Source: CAD feature listing. Evaluate the final solid. Frame: model axes, mm. A direction names the side the tool comes from. Coordinates: 2 decimals unless noted, no trailing zeros. Order: outer loops, then holes, each group sorted by start corner. A loop starts at its lowest first (then second) coordinate and runs counter-clockwise, first axis right, second up. Notation, with made-up numbers: (51.25, 58.5) -> (80.25, 58.5) arc R20 ccw to (80.25, 77.5) -> close; hole circle Ø6 at (24, 66). An arc over 180 degrees is marked (long way). Write item = value, one per line. Start each with the question number.
Item 1: Section query A-A (y = 24). Count the separate pieces of the cut face and the enclosed holes in it, then the cut area to 3 significant figures.
Item 2: Section query C-C (z = 11). Output: boundary loops of the cut face in (x, y), then the cut area to 3 significant figures.
Item 3: Section query D-D (x = 26). Output: boundary loops of the cut face in (y, z).
Item 4: Set-up query: faces 5 (the flat face through (58.234, 18.872, 42.555)), 6 (the cylindrical face through (-40.992, 1.565, -38.977)), 7 (the flat face through (70.94, 18.87, 19.01)), 8 (the flat face through (-70.94, 18.87, 19.01)). Return all of +Z, -Z, +X, -X, +Y, -Y with unobstructed straight access to the full face (end or side cutting, diameter ignored); none if empty.
Item 5: Contact query for flat-ended pins moving along their axis: pin 1 (12 mm diameter, centred on y = 10.5, z = 33.5, fed in from -X); pin 2 (10 mm diameter, centred on y = 7, z = -70.5, fed in from +X); pin 3 (6 mm diameter, centred on y = 13, z = 21, fed in from -X). Output: stop coordinate, or through.
Item 6: Ray query, line 1 along Z through (x, y) = (58, 13.5); line 2 along X through (y, z) = (4.65, 41.91); line 3 along Z through (x, y) = (-56, 11.5). Return the intervals inside material, ascending. Write a range as [from, to].
Item 7: Mould query, pull axis X, two halves, no side actions, for faces 1 (the flat face through (-57.4, 19.5, 46.5)), 2 (the flat face through (71.2, 31.75, -24.6)), 3 (the cylindrical face through (77.376, 18.872, -39.764)), 4 (the flat face through (70.94, 18.87, -19.01)). Classes: released by +X, released by -X, zero draft, split by the parting line, or undercut.
Item 8: Section query B-B (x = -2.5). Output: boundary loops of the cut face in (y, z).
```python
from build123d import *
from build123d.topology import SkipClean

# Parameters (mm, degrees)
SKETCH1_R                     = 89.535
SKETCH1_R_2                   = 53.975
BASE_DEPTH                    = 6.35
NOCE_START                    = -6.35
NOCE_CONE_PYROS_DEPTH         = 6.35
BATTERY_1_HOLDER_DEPTH        = 25.4
BATTERY_4_HOLDER_COPY_1_DEPTH = 25.4
BATTERY_4_HOLDER_COPY_2_DEPTH = 25.4
SKETCH4_R                     = 3.81
BOLT_HOLE_DEPTH               = 6.35
BOLT_HOLE_4_COPY_1_SKETCH_R   = 3.81
BOLT_HOLE_4_COPY_1_DEPTH      = 6.35
BOLT_HOLE_4_COPY_2_SKETCH_R   = 3.81
BOLT_HOLE_4_COPY_2_DEPTH      = 6.35
SKETCH11_R                    = 5.08
CUT_EXTRUDE2_DEPTH            = 6.35
SKETCH13_R                    = 3.175
CUT_EXTRUDE3_DEPTH            = 3.175
SKETCH14_R                    = 1.524
CUT_EXTRUDE4_DEPTH            = 3.175
FILLET3_R                     = 1.27
SKETCH15_R                    = 1.524
CUT_EXTRUDE5_DEPTH            = 6.35


with BuildPart() as part:
    # Sketch1 → Base (new body)
    with BuildSketch(Plane(origin=(0, 0, 0), x_dir=(1, 0, 0), z_dir=(0, 1, 0))):
        with Locations(Location((0, 0, 0), (0, 0, 270))):
            Circle(SKETCH1_R)
        with Locations(Location((0, 0, 0), (0, 0, 270))):
            Circle(SKETCH1_R_2, mode=Mode.SUBTRACT)
    extrude(amount=BASE_DEPTH)

    # Sketch2 → Noce Cone Pyros (cut)
    with BuildSketch(Plane(origin=(0, 6.35, 0), x_dir=(1, 0, 0), z_dir=(0, 1, 0)).offset(NOCE_START)):
        with BuildLine():
            Line((89.3564, 5.652439), (88.3404, 5.652439))
            ThreePointArc((88.3404, 5.652439), (61.595, 0), (88.3404, -5.652439))
            Line((88.3404, -5.652439), (89.3564, -5.652439))
            ThreePointArc((89.3564, -5.652439), (89.490339, -2.82763), (89.535, 0))
            ThreePointArc((89.535, 0), (89.490339, 2.82763), (89.3564, 5.652439))
        make_face()
    noce_cone_pyros = extrude(amount=NOCE_CONE_PYROS_DEPTH, mode=Mode.SUBTRACT)

    # Nose Cone Pyro mirror: Noce Cone Pyros across plane
    add(noce_cone_pyros.mirror(Plane(origin=(0, 0, 0), x_dir=(0, 0, 1), z_dir=(1, 0, 0))), mode=Mode.SUBTRACT)

    # Sketch3 → Battery 1 Holder (add)
    with BuildSketch(Plane(origin=(0, 6.35, 0), x_dir=(1, 0, 0), z_dir=(0, 1, 0))):
        with BuildLine():
            ThreePointArc((55.138033, 17.288828), (55.489291, 16.125907), (55.816024, 14.955859))
            Line((55.816024, 14.955859), (86.484169, 23.173363))
            ThreePointArc((86.484169, 23.173363), (80.316454, 39.569982), (71.074049, 54.451775))
            Line((71.074049, 54.451775), (43.281478, 38.286027))
            ThreePointArc((43.281478, 38.286027), (44.112475, 37.325538), (44.922161, 36.347018))
            Line((44.922161, 36.347018), (71.924647, 48.938484))
            ThreePointArc((71.924647, 48.938484), (77.444747, 39.628792), (81.766133, 29.705715))
            Line((81.766133, 29.705715), (55.138033, 17.288828))
        make_face()
    battery_1_holder = extrude(amount=BATTERY_1_HOLDER_DEPTH)

    # Batery 2 Holder: Battery 1 Holder across plane
    add(battery_1_holder.mirror(Plane.XY))

    # Battery 3 Holder: Battery 1 Holder across plane
    with SkipClean():  # the faces are left unmerged after this step: merging them gives an invalid solid
        add(battery_1_holder.mirror(Plane(origin=(0, 0, 0), x_dir=(0, 0, 1), z_dir=(1, 0, 0))))

    # Battery 4 Holder copy 1 sketch → Battery 4 Holder copy 1 (add)
    with SkipClean():  # the faces are left unmerged after this step: merging them gives an invalid solid
        with BuildSketch(Plane(origin=(0, 6.35, 0), x_dir=(-1, 0, 0), z_dir=(0, 1, 0))):
            with BuildLine():
                ThreePointArc((55.138033, 17.288828), (55.489291, 16.125907), (55.816024, 14.955859))
                Line((55.816024, 14.955859), (86.484169, 23.173363))
                ThreePointArc((86.484169, 23.173363), (80.316454, 39.569982), (71.074049, 54.451775))
                Line((71.074049, 54.451775), (43.281478, 38.286027))
                ThreePointArc((43.281478, 38.286027), (44.112475, 37.325538), (44.922161, 36.347018))
                Line((44.922161, 36.347018), (71.924647, 48.938484))
                ThreePointArc((71.924647, 48.938484), (77.444747, 39.628792), (81.766133, 29.705715))
                Line((81.766133, 29.705715), (55.138033, 17.288828))
            make_face()
        extrude(amount=BATTERY_4_HOLDER_COPY_1_DEPTH)

    # Battery 4 Holder copy 2 sketch → Battery 4 Holder copy 2 (add)
    with SkipClean():  # the faces are left unmerged after this step: merging them gives an invalid solid
        with BuildSketch(Plane(origin=(0, 6.35, 0), x_dir=(-1, 0, 0), z_dir=(0, 1, 0))):
            with BuildLine():
                ThreePointArc((55.138033, -17.288828), (55.489291, -16.125907), (55.816024, -14.955859))
                Line((55.816024, -14.955859), (86.484169, -23.173363))
                ThreePointArc((86.484169, -23.173363), (80.316454, -39.569982), (71.074049, -54.451775))
                Line((71.074049, -54.451775), (43.281478, -38.286027))
                ThreePointArc((43.281478, -38.286027), (44.112475, -37.325538), (44.922161, -36.347018))
                Line((44.922161, -36.347018), (71.924647, -48.938484))
                ThreePointArc((71.924647, -48.938484), (77.444747, -39.628792), (81.766133, -29.705715))
                Line((81.766133, -29.705715), (55.138033, -17.288828))
            make_face()
        extrude(amount=BATTERY_4_HOLDER_COPY_2_DEPTH)

    # Sketch4 → Bolt Hole (cut)
    with SkipClean():  # the faces are left unmerged after this step: merging them gives an invalid solid
        with BuildSketch(Plane(origin=(0, 6.35, 0), x_dir=(1, 0, 0), z_dir=(0, 1, 0))):
            with Locations(Location((38.1, 65.991136, 0), (0, 0, 270))):
                Circle(SKETCH4_R)
        bolt_hole = extrude(amount=-BOLT_HOLE_DEPTH, mode=Mode.SUBTRACT)

    # Bolt Hole 2: Bolt Hole across plane
    with SkipClean():  # the faces are left unmerged after this step: merging them gives an invalid solid
        add(bolt_hole.mirror(Plane.XY), mode=Mode.SUBTRACT)

    # Bolt Hole 3: Bolt Hole across plane
    with SkipClean():  # the faces are left unmerged after this step: merging them gives an invalid solid
        add(bolt_hole.mirror(Plane(origin=(0, 0, 0), x_dir=(0, 0, 1), z_dir=(1, 0, 0))), mode=Mode.SUBTRACT)

    # Bolt Hole 4 copy 1 sketch → Bolt Hole 4 copy 1 (cut)
    with SkipClean():  # the faces are left unmerged after this step: merging them gives an invalid solid
        with BuildSketch(Plane(origin=(0, 6.35, 0), x_dir=(-1, 0, 0), z_dir=(0, 1, 0))):
            with Locations(Location((38.1, 65.991136, 0), (0, 0, 270))):
                Circle(BOLT_HOLE_4_COPY_1_SKETCH_R)
        extrude(amount=-BOLT_HOLE_4_COPY_1_DEPTH, mode=Mode.SUBTRACT)

    # Bolt Hole 4 copy 2 sketch → Bolt Hole 4 copy 2 (cut)
    with SkipClean():  # the faces are left unmerged after this step: merging them gives an invalid solid
        with BuildSketch(Plane(origin=(0, 6.35, 0), x_dir=(-1, 0, 0), z_dir=(0, 1, 0))):
            with Locations((38.1, -65.991136)):
                Circle(BOLT_HOLE_4_COPY_2_SKETCH_R)
        extrude(amount=-BOLT_HOLE_4_COPY_2_DEPTH, mode=Mode.SUBTRACT)

    # Sketch11 → Cut-Extrude2 (cut)
    with SkipClean():  # the faces are left unmerged after this step: merging them gives an invalid solid
        with BuildSketch(Plane.XZ):
            with Locations(Location((9.128366, 61.145977, 0), (0, 0, 270))):
                Circle(SKETCH11_R)
            with Locations(Location((-26.059706, 57.209264, 0), (0, 0, 270))):
                Circle(SKETCH11_R)
        extrude(amount=-CUT_EXTRUDE2_DEPTH, mode=Mode.SUBTRACT)

    # Sketch13 → Cut-Extrude3 (cut)
    with SkipClean():  # the faces are left unmerged after this step: merging them gives an invalid solid
        with BuildSketch(Plane.XZ):
            with Locations(Location((39.7764, 41.91, 0), (0, 0, 270))):
                Circle(SKETCH13_R)
            with Locations(Location((-39.7764, 41.91, 0), (0, 0, 270))):
                Circle(SKETCH13_R)
        cut_extrude3 = extrude(amount=-CUT_EXTRUDE3_DEPTH, mode=Mode.SUBTRACT)

    # Sketch14 → Cut-Extrude4 (cut)
    with SkipClean():  # the faces are left unmerged after this step: merging them gives an invalid solid
        with BuildSketch(Plane.XZ.offset(-3.175)):
            with Locations(Location((39.7764, 41.91, 0), (0, 0, 270))):
                Circle(SKETCH14_R)
            with Locations(Location((-39.7764, 41.91, 0), (0, 0, 270))):
                Circle(SKETCH14_R)
        cut_extrude4 = extrude(amount=-CUT_EXTRUDE4_DEPTH, mode=Mode.SUBTRACT)

    # Mirror1: Cut-Extrude3, Cut-Extrude4 across plane
    with SkipClean():  # the faces are left unmerged after this step: merging them gives an invalid solid
        add(cut_extrude3.mirror(Plane.XY), mode=Mode.SUBTRACT)
        add(cut_extrude4.mirror(Plane.XY), mode=Mode.SUBTRACT)

    # Fillet3
    # the kernel refuses this fillet: 1.27 mm, written as the material it adds along each edge
    with BuildSketch(Plane(origin=(-73.818547, 6.35, 56.048132), x_dir=(0.5027895932474892, 0, 0.8644088297339543), z_dir=(0.8644088297339544, 0, -0.5027895932474892))) as fillet3_piece_1_section:
        with BuildLine():
            CenterArc((FILLET3_R, -FILLET3_R), FILLET3_R, 90, 90)
            Line((0, -FILLET3_R), (0, 0))
            Line((0, 0), (FILLET3_R, 0))
        make_face()
    fillet3_piece_1 = extrude(amount=38.502113, mode=Mode.PRIVATE)
    fillet3_piece_1 = fillet3_piece_1 & Plane(origin=(0, 6.637419, 0), x_dir=(0, 0, 1), z_dir=(0, -1, 0)) * Cylinder(89.535, 83, mode=Mode.PRIVATE)
    fillet3_piece_1 = fillet3_piece_1 - Plane(origin=(0, 6.637419, 0), x_dir=(-0.7490088761778874, 0, 0.6625599621217225), z_dir=(0, -1, 0)) * Cylinder(57.785, 83, mode=Mode.PRIVATE)
    add(fillet3_piece_1)
    with BuildSketch(Plane(origin=(73.818547, 6.35, -56.048132), x_dir=(-0.5027895932474892, 0, -0.8644088297339543), z_dir=(-0.8644088297339544, 0, 0.5027895932474892))) as fillet3_piece_2_section:
        with BuildLine():
            CenterArc((FILLET3_R, -FILLET3_R), FILLET3_R, 90, 90)
            Line((0, -FILLET3_R), (0, 0))
            Line((0, 0), (FILLET3_R, 0))
        make_face()
    fillet3_piece_2 = extrude(amount=38.502113, mode=Mode.PRIVATE)
    fillet3_piece_2 = fillet3_piece_2 - Plane(origin=(0, 6.637419, 0), x_dir=(0.7490088761778874, 0, -0.6625599621217225), z_dir=(0, -1, 0)) * Cylinder(57.785, 83, mode=Mode.PRIVATE)
    fillet3_piece_2 = fillet3_piece_2 & Plane(origin=(0, 6.637419, 0), x_dir=(0, 0, 1), z_dir=(0, -1, 0)) * Cylinder(89.535, 83, mode=Mode.PRIVATE)
    add(fillet3_piece_2)
    with BuildSketch(Plane(origin=(73.818547, 6.35, 56.048132), x_dir=(-0.5027895932474892, 0, 0.8644088297339543), z_dir=(-0.8644088297339544, 0, -0.5027895932474892))) as fillet3_piece_3_section:
        with BuildLine():
            CenterArc((FILLET3_R, FILLET3_R), FILLET3_R, 180, 90)
            Line((0, FILLET3_R), (0, 0))
            Line((0, 0), (FILLET3_R, 0))
        make_face()
    fillet3_piece_3 = extrude(amount=38.502113, mode=Mode.PRIVATE)
    fillet3_piece_3 = fillet3_piece_3 & Plane(origin=(0, 6.637418, 0), x_dir=(0, 0, 1), z_dir=(0, -1, 0)) * Cylinder(89.535, 83, mode=Mode.PRIVATE)
    fillet3_piece_3 = fillet3_piece_3 - Plane(origin=(0, 6.637418, 0), x_dir=(0.7490088761778874, 0, 0.6625599621217225), z_dir=(0, -1, 0)) * Cylinder(57.785, 83, mode=Mode.PRIVATE)
    add(fillet3_piece_3)
    with BuildSketch(Plane(origin=(-73.818547, 6.35, -56.048132), x_dir=(0.5027895932474892, 0, -0.8644088297339543), z_dir=(0.8644088297339544, 0, 0.5027895932474892))) as fillet3_piece_4_section:
        with BuildLine():
            CenterArc((FILLET3_R, FILLET3_R), FILLET3_R, 180, 90)
            Line((0, FILLET3_R), (0, 0))
            Line((0, 0), (FILLET3_R, 0))
        make_face()
    fillet3_piece_4 = extrude(amount=38.502113, mode=Mode.PRIVATE)
    fillet3_piece_4 = fillet3_piece_4 & Plane(origin=(0, 6.637418, 0), x_dir=(0, 0, 1), z_dir=(0, -1, 0)) * Cylinder(89.535, 83, mode=Mode.PRIVATE)
    fillet3_piece_4 = fillet3_piece_4 - Plane(origin=(0, 6.637418, 0), x_dir=(-0.7490088761778874, 0, -0.6625599621217225), z_dir=(0, -1, 0)) * Cylinder(57.785, 83, mode=Mode.PRIVATE)
    add(fillet3_piece_4)

    # Sketch15 → Cut-Extrude5 (cut)
    with BuildSketch(Plane.XZ):
        with Locations(Location((57.785, 0, 0), (0, 0, 270))):
            Circle(SKETCH15_R)
    cut_extrude5 = extrude(amount=-CUT_EXTRUDE5_DEPTH, mode=Mode.SUBTRACT)

    # Mirror2: Cut-Extrude5 across plane
    add(cut_extrude5.mirror(Plane(origin=(0, 0, 0), x_dir=(0, 0, 1), z_dir=(1, 0, 0))), mode=Mode.SUBTRACT)


solid = part.part
```
Computed:
q1.separate_pieces = 4
q1.enclosed_holes = 0
q1.area = 1,390 mm^2
q2.outline = (-88.86, 0) -> (-84.18, 0) -> (-84.18, 6.35) -> (-88.86, 6.35) -> close; (-66.95, 0) -> (-52.84, 0) -> (-52.84, 6.35) -> (-66.95, 6.35) -> close; (52.84, 0) -> (66.95, 0) -> (66.95, 6.35) -> (52.84, 6.35) -> close; (84.18, 0) -> (88.86, 0) -> (88.86, 6.35) -> (84.18, 6.35) -> close
q2.area = 239 mm^2
q3.outline = (0, -85.68) -> (6.35, -85.68) -> (6.35, -47.3) -> (0, -47.3) -> close; (0, 47.3) -> (6.35, 47.3) -> (6.35, 85.68) -> (0, 85.68) -> close
q4.face_5 = +Y
q4.face_6 = -Y
q4.face_7 = +X, +Y
q4.face_8 = -X, +Y
q5.pin_1 = -85.21
q5.pin_2 = 61
q5.pin_3 = -86.48
q6.line_1 = [-46.85, -42.45], [-18.62, -15.54], [15.54, 18.62], [42.45, 46.85]
q6.line_2 = [-79.12, -41.3], [-38.25, -34.01], [34.01, 38.25], [41.3, 79.12]
q6.line_3 = [-45.68, -41.51], [-17.69, -15.01], [15.01, 17.69], [41.51, 45.68]
q7.face_1 = undercut
q7.face_2 = zero draft
q7.face_3 = undercut
q7.face_4 = released by +X
q8.outline = (0, -89.5) -> (6.35, -89.5) -> (6.35, -53.92) -> (0, -53.92) -> close; (0, 53.92) -> (6.35, 53.92) -> (6.35, 89.5) -> (0, 89.5) -> close
